The figure shows three views and two pictorial views of one solid part (mm, origin at its lowest corner). Answer the questions. A direction names the side the tool comes from. Give positions to 0.01 mm unless a question says otherwise; leave off trailing zeros. Loops run counter-clockwise (first coordinate to the right, second up) from the corner with the lowest first, then second, coordinate; pieces in that order, holes last.
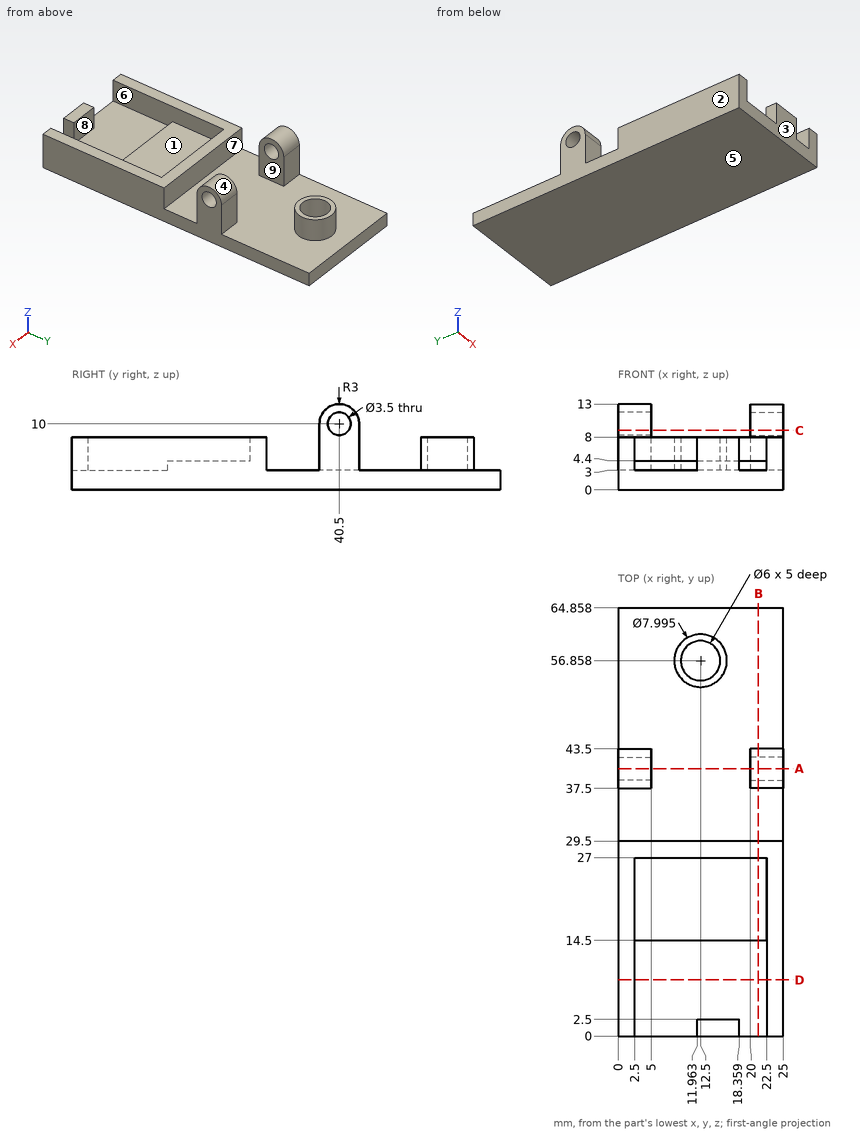
Q1. Section C-C on z = 9 is taken. Give the vertices of the cut face in (x, y).
Q2. Section A-A on y = 40.5 is taken. Give the vertices of the cut face in (x, z).
Q3. Which of the six approach directions +Z, -Z, +X, -X, +Y, -Y give full straight-line access (tool end or side, diameter ignored) to the marked faces 5, 6, 7, 8 and 9?
Q4. Determine the mould class of the marked faces 1, 2, 3 and 4 for opening direction Y: +Y half, -Y half, draft (parallel to the pull), parting line (faces both ways), or undercut.
Q5. Section B-B on x = 21.25 is taken. Give the vertices of the cut face in (y, z), plus the area to 3 significant figures.
Q6. Section D-D on y = 8.5 is taken. Give the vertices of the cut face in (x, z), plus the area to 3 significant figures.
Q7. Given pin 1 (2 mm diameter, centred on y = 56.5, z = 8, fed in from -X); pin 2 (6 mm diameter, centred on x = 16, y = 21.5, fed in from +Z); pin 3 (1.2 mm diameter, centred on x = 14.5, y = 1.5, fed in from +Z), each flat-ended and moving along its own axis, determine where each tip first touches the part or whether it passes through.
Q8. Consider line 1 along Y through (x, z) = (21.6, 10); line 2 along Y through (x, z) = (12.5, 5.55) (1 decimal); line 3 along Z through (x, y) = (3.05, 40.5). Determine where each line is inside the solid, lowest interval first.
Check result:
1. outline: (0, 37.5) - (5, 37.5) - (5, 39.06) - (0, 39.06) - close; (0, 41.94) - (5, 41.94) - (5, 43.5) - (0, 43.5) - close; (20, 37.5) - (25, 37.5) - (25, 39.06) - (20, 39.06) - close; (20, 41.94) - (25, 41.94) - (25, 43.5) - (20, 43.5) - close
2. outline: (0, 0) - (25, 0) - (25, 8.25) - (20, 8.25) - (20, 3) - (5, 3) - (5, 8.25) - (0, 8.25) - close; (0, 11.75) - (5, 11.75) - (5, 13) - (0, 13) - close; (20, 11.75) - (25, 11.75) - (25, 13) - (20, 13) - close
3. face 5: -Z, +X, -X, +Y, -Y
3. face 6: +Z, -Y
3. face 7: +Z, +X, -X
3. face 8: +Z
3. face 9: +Z, +Y
4. face 1: undercut
4. face 2: draft
4. face 3: -Y half
4. face 4: parting line
5. outline: (0, 0) - (64.86, 0) - (64.86, 3) - (43.5, 3) - (43.5, 10) arc R3 ccw to (37.5, 10) - (37.5, 3) - (29.5, 3) - (29.5, 8) - (27, 8) - (27, 4.4) - (14.5, 4.4) - (14.5, 3) - (0, 3) - close; hole circle Ø3.5 at (40.5, 10)
5. area: 271 mm2
6. outline: (0, 0) - (25, 0) - (25, 8) - (22.5, 8) - (22.5, 3) - (2.5, 3) - (2.5, 8) - (0, 8) - close
6. area: 100 mm2
7. pin 1: stops at x = 8.5
7. pin 2: stops at z = 4.4
7. pin 3: stops at z = 8
8. line 1: y = 37.5 to 38.75, 42.25 to 43.5
8. line 2: y = 0 to 2.5, 27 to 29.5, 52.9 to 53.9, 59.9 to 60.9
8. line 3: z = 0 to 8.25, 11.75 to 13
